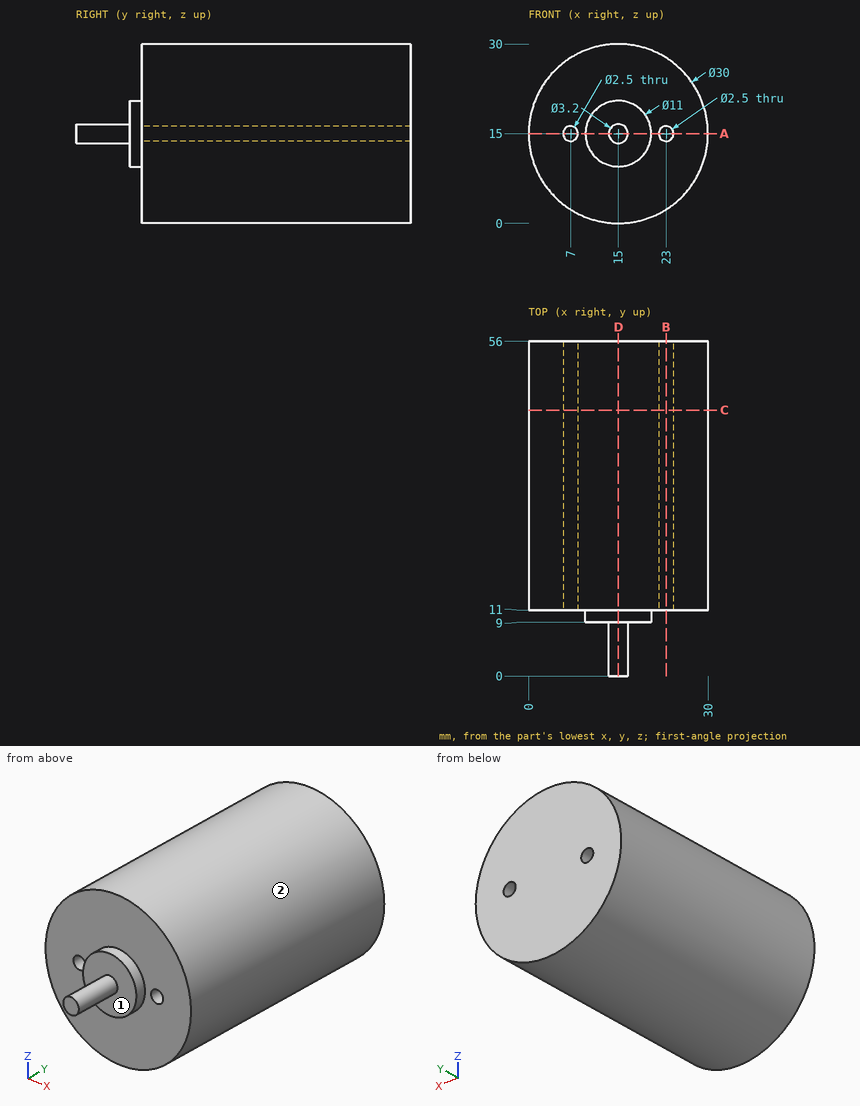
Input: dimensioned drawing with shaded views. Units: mm. Origin: part minimum x, y, z. A direction names the side the tool comes from. Round coordinates to 2 decimals unless told otherwise and drop trailing zeros. Order: outer loops, then holes, each group sorted by start corner. A loop starts at its lowest first (then second) coordinate and runs counter-clockwise, first axis right, second up.
1. Cut plane C-C, the plane y = 44.5. Output: boundary loops of the cut face in (x, z).
The answers:
outline: circle Ø30 at (15, 15); hole circle Ø2.5 at (7, 15); hole circle Ø2.5 at (23, 15)
2. Cut plane D-D, the plane x = 15. Output: boundary loops of the cut face in (y, z), then the cut area to 3 significant figures.
The answers:
outline: (0, 13.4) - (9, 13.4) - (9, 9.5) - (11, 9.5) - (11, 0) - (56, 0) - (56, 30) - (11, 30) - (11, 20.5) - (9, 20.5) - (9, 16.6) - (0, 16.6) - close
area: 1,400 mm2
3. Cut plane A-A, the plane z = 15. Output: boundary loops of the cut face in (x, y).
The answers:
outline: (0, 11) - (5.75, 11) - (5.75, 56) - (0, 56) - close; (8.25, 11) - (9.5, 11) - (9.5, 9) - (13.4, 9) - (13.4, 0) - (16.6, 0) - (16.6, 9) - (20.5, 9) - (20.5, 11) - (21.75, 11) - (21.75, 56) - (8.25, 56) - close; (24.25, 11) - (30, 11) - (30, 56) - (24.25, 56) - close
4. Material intervals for line 1 (Y direction, x = 15.75, z = 21); line 2 (Z direction, x = 7, y = 20); line 3 (Z direction, x = 15, y = 46.5), sorted ascending.
The answers:
line 1: y = 11 to 56
line 2: z = 2.31 to 13.75, 16.25 to 27.69
line 3: z = 0 to 30
5. Set-up query: the marked faces 1 and 2. Return all of +Z, -Z, +X, -X, +Y, -Y with unobstructed straight access to the full face (end or side cutting, diameter ignored); none if empty.
The answers:
face 1: -Y
face 2: +Y, -Y
6. Cut plane B-B, the plane x = 23. Output: boundary loops of the cut face in (y, z).
The answers:
outline: (11, 2.31) - (56, 2.31) - (56, 13.75) - (11, 13.75) - close; (11, 16.25) - (56, 16.25) - (56, 27.69) - (11, 27.69) - close
7. Pin query (flat end, axial travel): P1, Ø2, axis at y = 43.5, z = 24.5, coming from the +X side; P2, Ø4, axis at x = 5.5, y = 20, coming from the +Z side; P3, Ø1.5, axis at x = 26, z = 7.5, coming from the -Y side. Return the tip coordinate at first contact, or that it passes through.
The answers:
P1: stops at x = 27.36
P2: stops at z = 27.99
P3: stops at y = 11
